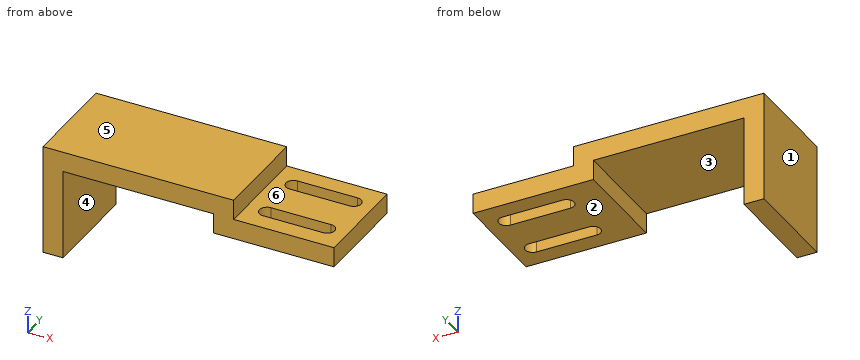
from build123d import *

# Parameters (mm, degrees)
SALIENTE_EXTRUIR1_DEPTH = 20
CORTAR_EXTRUIR1_DEPTH   = 20


with BuildPart() as part:
    # Croquis1 → Saliente-Extruir1 (new body)
    with BuildSketch(Plane(origin=(0, 0, 0), x_dir=(1, 0, 0), z_dir=(0, 1, 0))):
        Polygon((-19, 22), (-15, 22), (-15, 4), (15, 4), (15, 8), (39, 8), (39, 4), (19, 4), (19, 0), (-19, 0), align=None)
    extrude(amount=SALIENTE_EXTRUIR1_DEPTH)

    # Croquis2 → Cortar-Extruir1 (cut)
    with BuildSketch(Plane.XY.offset(-4)):
        with BuildLine():
            Line((35, 16.5), (23, 16.5))
            ThreePointArc((23, 16.5), (21.5, 15), (23, 13.5))
            Line((23, 13.5), (35, 13.5))
            ThreePointArc((35, 13.5), (36.5, 15), (35, 16.5))
        make_face()
        with BuildLine():
            Line((35, 3.5), (23, 3.5))
            ThreePointArc((23, 3.5), (21.5, 5), (23, 6.5))
            Line((23, 6.5), (35, 6.5))
            ThreePointArc((35, 6.5), (36.5, 5), (35, 3.5))
        make_face()
    extrude(amount=-CORTAR_EXTRUIR1_DEPTH, mode=Mode.SUBTRACT)


solid = part.part
Input: part model. Units: mm. Frame: model coordinates. Face numbers are marked on the shaded views. A direction names the side the tool comes from. Give positions to 0.01 mm unless a question says otherwise; leave off trailing zeros. Loops run counter-clockwise (first coordinate to the right, second up) from the corner with the lowest first, then second, coordinate; pieces in that order, holes last. Notation, with made-up numbers: M 35,-26.5 L 93,-26.5 A16 ccw 93,0.5 Z; hole C -6,88.5 d7. An arc over 180 degrees is marked long. Use one line per item in the form item = value.
1. First-contact query: pin 1 (5.5 mm diameter, centred on y = 10, z = -12, fed in from +X); pin 2 (6 mm diameter, centred on x = 28, y = 7, fed in from +Z); pin 3 (2 mm diameter, centred on x = -4, y = 17.5, fed in from -Z). Flat tips, straight axial feed; report the tip coordinate or a pass-through.
Numbers:
pin_1 = -15
pin_2 = -4
pin_3 = -4
2. Section query D-D, the plane y = 9. Return the cut outline in (x, z), and give its area (3 significant figures).
Numbers:
outline = M -19,-22 L -15,-22 L -15,-4 L 15,-4 L 15,-8 L 39,-8 L 39,-4 L 19,-4 L 19,0 L -19,0 Z
area = 320 mm²
3. Reachability of the marked faces 5 and 6 from +Z, -Z, +X, -X, +Y, -Y: full face, straight path, thin tool, end or side. Return the list, or none.
Numbers:
face_5 = +Z, +X, -X, +Y, -Y
face_6 = +Z, +X, +Y, -Y
4. Section query C-C, the plane y = 5. Return the cut outline in (x, z), and give its area (3 significant figures).
Numbers:
outline = M -19,-22 L -15,-22 L -15,-4 L 15,-4 L 15,-8 L 21.5,-8 L 21.5,-4 L 19,-4 L 19,0 L -19,0 Z; M 36.5,-8 L 39,-8 L 39,-4 L 36.5,-4 Z
area = 260 mm²
5. Pull-direction query (X, two-part tool) for the marked faces 1, 2, 3 and 4; classes: released by +X, released by -X, zero draft, split by the parting line, or undercut.
Numbers:
face_1 = released by -X
face_2 = zero draft
face_3 = undercut
face_4 = undercut
6. Section query B-B, the plane x = 31.5. Return the cut outline in (y, z), and give its area (3 significant figures).
Numbers:
outline = M 0,-8 L 3.5,-8 L 3.5,-4 L 0,-4 Z; M 6.5,-8 L 13.5,-8 L 13.5,-4 L 6.5,-4 Z; M 16.5,-8 L 20,-8 L 20,-4 L 16.5,-4 Z
area = 56.0 mm²
7. Section query A-A, the plane z = -5.5. Return the cut outline in (x, y), and give its area (3 significant figures).
Numbers:
outline = M -19,0 L -15,0 L -15,20 L -19,20 Z; M 15,0 L 39,0 L 39,20 L 15,20 Z; hole M 23,3.5 L 35,3.5 A1.5 ccw 35,6.5 L 23,6.5 A1.5 ccw Z; hole M 23,13.5 L 35,13.5 A1.5 ccw 35,16.5 L 23,16.5 A1.5 ccw Z
area = 474 mm²
8. Line query: L1, parallel to Y at x = 30, z = -6; L2, parallel to X at y = 3.75, z = -5.75; L3, parallel to X at y = 16.75, z = -7.75. Output: solid intervals per line, ascending.
Numbers:
L1 = 0 to 3.5, 6.5 to 13.5, 16.5 to 20
L2 = -19 to -15, 15 to 22.17, 35.83 to 39
L3 = -19 to -15, 15 to 39
